```python
from build123d import *

# Parameters (mm, degrees)
PAD_DEPTH       = 30
SKETCH003_R     = 5
HOLE_DEPTH      = 44
HOLE_TIPS_R     = 5
SKETCH005_R     = 2.5
HOLE001_DEPTH   = 60.001
SKETCH011_R     = 3.2
HOLE002_DEPTH   = 60
HOLE002_TIPS_R  = 3.2
SKETCH013_R     = 1.25
HOLE003_DEPTH   = 10
HOLE003_TIPS_R  = 1.25
SKETCH014_R     = 3.4
HOLE004_DEPTH   = 20
HOLE004_TIPS_R  = 3.4
SKETCH015_R     = 10
SKETCH015_R_2   = 3.5
SKETCH015_W     = 112.5
SKETCH015_H     = 5
POCKET001_DEPTH = 5
SKETCH016_R     = 1.6
HOLE005_DEPTH   = 20
HOLE005_TIPS_R  = 1.6
SKETCH029_R     = 2.5
POCKET007_DEPTH = 60.001


with BuildPart() as part:
    # Sketch → Revolution (revolve)
    with BuildSketch(Plane.XZ):
        Polygon((6, 60), (6.75, 30), (0, 30), (0, 60), align=None)
    revolve(axis=Axis((0, 0, 0), (0, 0, 1)))

    # Sketch006 → Pad (new body)
    with BuildSketch(Plane.XY):
        Polygon((0, 17.5), (62.5, 17.5), (62.5, -17.5), (0, -17.5), (-17.5, -17.5), (-17.5, 17.5), align=None)
    extrude(amount=PAD_DEPTH)

    # Sketch003 → Hole (cut)
    with BuildSketch(Plane.XY.offset(60)):
        Circle(SKETCH003_R)
    extrude(amount=-HOLE_DEPTH, mode=Mode.SUBTRACT)

    # Hole tips → Hole tip 1 section 0
    with BuildSketch(Plane.XY.offset(16), mode=Mode.PRIVATE) as hole_tip_1_s0:
        Circle(HOLE_TIPS_R)
    loft([hole_tip_1_s0.sketch, Vertex(0, 0, 12.995697)], mode=Mode.SUBTRACT)

    # Sketch005 → Hole001 (cut, through all)
    with BuildSketch(Plane.XY):
        with Locations((-2.5, 0)):
            Circle(SKETCH005_R)
    extrude(amount=HOLE001_DEPTH, mode=Mode.SUBTRACT)

    # Sketch011 → Hole002 (cut)
    with BuildSketch(Plane.YZ.offset(62.5)):
        with Locations((0, 20)):
            Circle(SKETCH011_R)
    extrude(amount=-HOLE002_DEPTH, mode=Mode.SUBTRACT)

    # Hole002 tips → Hole002 tip 1 section 0
    with BuildSketch(Plane.YZ.offset(2.5), mode=Mode.PRIVATE) as hole002_tip_1_s0:
        with Locations((0, 20)):
            Circle(HOLE002_TIPS_R)
    loft([hole002_tip_1_s0.sketch, Vertex(0.577246, 0, 20)], mode=Mode.SUBTRACT)

    # Sketch012 → Groove (revolve, cut)
    with BuildSketch(Plane.YZ.offset(45)):
        Polygon((15, 30), (15, 29), (12.9, 29), (12.9, 27.5), (10.4, 27.5), (10.4, 27.9), (10, 27.9), (10, 11.5), (5.4, 11.5), (4.788889, 6.5), (2.5, 6.5), (2.5, 0), (0, 0), (0, 30), align=None)
    revolve(axis=Axis((45, 0, 0), (0, 0, 1)), mode=Mode.SUBTRACT)

    # Sketch013 → Hole003 (cut)
    with BuildSketch(Plane.XY.offset(30)):
        with Locations((33.25, 13.75)):
            Circle(SKETCH013_R)
        with Locations((56.75, 13.75)):
            Circle(SKETCH013_R)
        with Locations((33.25, -13.75)):
            Circle(SKETCH013_R)
        with Locations((56.75, -13.75)):
            Circle(SKETCH013_R)
    extrude(amount=-HOLE003_DEPTH, mode=Mode.SUBTRACT)

    # Hole003 tips → Hole003 tip 1 section 0
    with BuildSketch(Plane.XY.offset(20), mode=Mode.PRIVATE) as hole003_tip_1_s0:
        with Locations((33.25, 13.75)):
            Circle(HOLE003_TIPS_R)
    loft([hole003_tip_1_s0.sketch, Vertex(33.25, 13.75, 19.248924)], mode=Mode.SUBTRACT)

    # Hole003 tips → Hole003 tip 2 section 0
    with BuildSketch(Plane.XY.offset(20), mode=Mode.PRIVATE) as hole003_tip_2_s0:
        with Locations((56.75, 13.75)):
            Circle(HOLE003_TIPS_R)
    loft([hole003_tip_2_s0.sketch, Vertex(56.75, 13.75, 19.248924)], mode=Mode.SUBTRACT)

    # Hole003 tips → Hole003 tip 3 section 0
    with BuildSketch(Plane.XY.offset(20), mode=Mode.PRIVATE) as hole003_tip_3_s0:
        with Locations((33.25, -13.75)):
            Circle(HOLE003_TIPS_R)
    loft([hole003_tip_3_s0.sketch, Vertex(33.25, -13.75, 19.248924)], mode=Mode.SUBTRACT)

    # Hole003 tips → Hole003 tip 4 section 0
    with BuildSketch(Plane.XY.offset(20), mode=Mode.PRIVATE) as hole003_tip_4_s0:
        with Locations((56.75, -13.75)):
            Circle(HOLE003_TIPS_R)
    loft([hole003_tip_4_s0.sketch, Vertex(56.75, -13.75, 19.248924)], mode=Mode.SUBTRACT)

    # Sketch014 → Hole004 (cut)
    with BuildSketch(Plane.YZ.offset(62.5)):
        with Locations((0, 20)):
            Circle(SKETCH014_R)
    extrude(amount=-HOLE004_DEPTH, mode=Mode.SUBTRACT)

    # Hole004 tips → Hole004 tip 1 section 0
    with BuildSketch(Plane.YZ.offset(42.5), mode=Mode.PRIVATE) as hole004_tip_1_s0:
        with Locations((0, 20)):
            Circle(HOLE004_TIPS_R)
    loft([hole004_tip_1_s0.sketch, Vertex(40.457074, 0, 20)], mode=Mode.SUBTRACT)

    # Sketch015 → Pocket001 (cut)
    with BuildSketch(Plane.XY.offset(4.5)):
        with Locations((45, 0)):
            Circle(SKETCH015_R)
        with Locations((45, 0)):
            Circle(SKETCH015_R_2, mode=Mode.SUBTRACT)
        with Locations((6.25, 15)):
            Rectangle(SKETCH015_W, SKETCH015_H)
        with Locations((6.25, -15)):
            Rectangle(SKETCH015_W, SKETCH015_H)
    extrude(amount=-POCKET001_DEPTH, mode=Mode.SUBTRACT)

    # Sketch016 → Hole005 (cut)
    with BuildSketch(Plane.YZ.offset(62.5)):
        with Locations((-12.5, 10)):
            Circle(SKETCH016_R)
        with Locations((12.5, 10)):
            Circle(SKETCH016_R)
    extrude(amount=-HOLE005_DEPTH, mode=Mode.SUBTRACT)

    # Hole005 tips → Hole005 tip 1 section 0
    with BuildSketch(Plane.YZ.offset(42.5), mode=Mode.PRIVATE) as hole005_tip_1_s0:
        with Locations((-12.5, 10)):
            Circle(HOLE005_TIPS_R)
    loft([hole005_tip_1_s0.sketch, Vertex(41.538623, -12.5, 10)], mode=Mode.SUBTRACT)

    # Hole005 tips → Hole005 tip 2 section 0
    with BuildSketch(Plane.YZ.offset(42.5), mode=Mode.PRIVATE) as hole005_tip_2_s0:
        with Locations((12.5, 10)):
            Circle(HOLE005_TIPS_R)
    loft([hole005_tip_2_s0.sketch, Vertex(41.538623, 12.5, 10)], mode=Mode.SUBTRACT)

    # Sketch029 → Pocket007 (cut, through all)
    with BuildSketch(Plane.XY):
        with Locations((25, 7.5)):
            Circle(SKETCH029_R)
    extrude(amount=POCKET007_DEPTH, mode=Mode.SUBTRACT)


solid = part.part
```
Geometry: final body of the model. Coordinates: model frame, mm. A direction names the side the tool comes from. Round coordinates to 2 decimals unless told otherwise and drop trailing zeros. Order: outer loops, then holes, each group sorted by start corner. A loop starts at its lowest first (then second) coordinate and runs counter-clockwise, first axis right, second up. Notation, with made-up numbers: (41, -6.75) - (56, -6.75) arc R17 cw to (56, 0.25) - close; hole circle Ø10 at (-20.75, -38.5). An arc over 180 degrees is marked (long way). Use CSV: the item, a comma, the result in double quotes. Start each with the question number.
Q1. Section query D-D (x = -8.5). Return loops of the section in (y, z).
Q2. Access query for faces 1 (the face through (49, 4, 11.5)), 2 (the face through (52.64, 10.9, 10.07)), 3 (the face through (43, -2, 0)), 4 (the face through (22, -15, 4.5)), 5 (the face through (22, 12.5, 2)). Directions: +Z, -Z, +X, -X, +Y, -Y. A direction counts if a zero-diameter tool reaches every point of the face in a straight line with its end or side. Return the directions, or none.
Q3. Section query A-A (x = 25). Return loops of the section in (y, z), and give its area (3 significant figures).
Q4. Section query C-C (x = 45). State how many separate pieces and enclosed holes the cut face has, and give its area (3 significant figures).
Q5. Mould query, pull axis X, two halves, no side actions, for faces 6 (the face through (57.94, -13.37, 25.07)), 7 (the face through (-1.38, -6.23, 44.79)), 8 (the face through (58.51, 3.14, 18.7)). Classes: +X half, -X half, draft (parallel to the pull), parting line (faces both ways), or undercut.
Q6. Material intervals for line 1 along Y through (x, z) = (45, 1.5); line 2 along Y through (x, z) = (33.25, 25.25); line 3 along X through (y, z) = (7.5, 24), sorted ascending. Write a range as from..to.
Q7. Section query B-B (z = 25.5). Return loops of the section in (x, y).
Q8. First-contact query: pin 1 (4 mm diameter, centred on x = 49.5, y = -3, fed in from +Z); pin 2 (6 mm diameter, centred on y = 0, z = 20, fed in from +X); pin 3 (5 mm diameter, centred on x = -4, z = 52.5, fed in from -Y). Flat tips, straight axial feed; report the tip coordinate or a pass-through.
Result set:
1,outline,"(-17.5, 4.5) - (-12.5, 4.5) - (-12.5, 0) - (12.5, 0) - (12.5, 4.5) - (17.5, 4.5) - (17.5, 30) - (-17.5, 30) - close"
2,face 1,"+Z"
2,face 2,"+X"
2,face 3,"-Z, +X, -X, +Y, -Y"
2,face 4,"-Z, +X, -X, -Y"
2,face 5,"-Z, +X, -X, +Y"
3,outline,"(-17.5, 4.5) - (-12.5, 4.5) - (-12.5, 0) - (5, 0) - (5, 30) - (-17.5, 30) - close; (10, 0) - (12.5, 0) - (12.5, 4.5) - (17.5, 4.5) - (17.5, 30) - (10, 30) - close; hole circle Ø6.4 at (0, 20)"
3,area,"823 mm2"
4,separate pieces,"2"
4,enclosed holes,"2"
4,area,"459 mm2"
5,face 6,"undercut"
5,face 7,"parting line"
5,face 8,"draft"
6,line 1,"y = -12.5..-10, -3.5..-2.5, 2.5..3.5, 10..12.5"
6,line 2,"y = -17.5..-15, -12.5..12.5, 15..17.5"
6,line 3,"x = -17.5..22.5, 27.5..38.39, 51.61..62.5"
7,outline,"(-17.5, -17.5) - (62.5, -17.5) - (62.5, 17.5) - (-17.5, 17.5) - close; hole circle Ø10 at (0, 0); hole circle Ø5 at (25, 7.5); hole circle Ø2.5 at (33.25, -13.75); hole circle Ø2.5 at (33.25, 13.75); hole circle Ø20 at (45, 0); hole circle Ø2.5 at (56.75, -13.75); hole circle Ø2.5 at (56.75, 13.75)"
8,pin 1,"stops at z = 11.5"
8,pin 2,"stops at x = -4"
8,pin 3,"stops at y = -6.01"
